Part model, mm, in its own coordinate system. Round coordinates to 2 decimals unless told otherwise and drop trailing zeros. Loops run counter-clockwise (first coordinate to the right, second up) from the corner with the lowest first, then second, coordinate; pieces in that order, holes last.
(1) Cut at A-A on z = 264.5. List the corners of the cut face in (x, y), then the cut area to 3 significant figures.
(2) Probe probe 1 along Y at (x, z) = (-6.9, 186); probe 2 along X at (y, z) = (-2.75, 123); probe 3 along X at (y, z) = (-3, 174.5). List the from-to ranges inside material, lowest first.
(3) Mould opens along X. For faces 1 (the face through (6, 4.95, 148)), 2 (the face through (0, -1.35, 148)), 3 (the face through (9.9, 0, 148)) say: +X half, -X half, draft (parallel to the pull), parting line (faces both ways), or undercut.
(4) Flat gauge pins, fed straight in: pin 1 (4 mm diameter, centred on x = 0, z = 125, fed in from +Y); pin 2 (0.5 mm diameter, centred on y = 5, z = 130, fed in from -X). Where does each tip first touch, or does it go through?
from build123d import *

# Parameters (mm, degrees)
SKETCH_1_R      = 2.1
EXTRUDE_1_DEPTH = 300


with BuildPart() as part:
    # 草图1 → 凸台-拉伸1 (new body)
    with BuildSketch(Plane.XY):
        with BuildLine():
            Line((8.4, -4.95), (-8.4, -4.95))
            ThreePointArc((-8.4, -4.95), (-9.460660172, -4.510660172), (-9.9, -3.45))
            Line((-9.9, -3.45), (-9.9, 3.45))
            ThreePointArc((-9.9, 3.45), (-9.460660172, 4.510660172), (-8.4, 4.95))
            Line((-8.4, 4.95), (-3.5, 4.95))
            Line((-3.5, 4.95), (-3.5, 4.338498403))
            Line((-3.5, 4.338498403), (-3.2, 4.338498403))
            Line((-3.2, 4.338498403), (-3.2, 3.15))
            Line((-3.2, 3.15), (-6.074788311, 3.15))
            Line((-6.074788311, 3.15), (-6.074788311, 0.842971246))
            Line((-6.074788311, 0.842971246), (-2.616641346, -1.35))
            Line((-2.616641346, -1.35), (2.616641346, -1.35))
            Line((2.616641346, -1.35), (6.074788311, 0.842971246))
            Line((6.074788311, 0.842971246), (6.074788311, 3.15))
            Line((6.074788311, 3.15), (3.2, 3.15))
            Line((3.2, 3.15), (3.2, 4.338498403))
            Line((3.2, 4.338498403), (3.5, 4.338498403))
            Line((3.5, 4.338498403), (3.5, 4.95))
            Line((3.5, 4.95), (8.4, 4.95))
            ThreePointArc((8.4, 4.95), (9.460660172, 4.510660172), (9.9, 3.45))
            Line((9.9, 3.45), (9.9, -3.45))
            ThreePointArc((9.9, -3.45), (9.460660172, -4.510660172), (8.4, -4.95))
        make_face()
        with Locations((-6.9, -1.95)):
            Circle(SKETCH_1_R, mode=Mode.SUBTRACT)
        with Locations(Location((6.9, -1.95, 0), (0, 0, 180))):
            Circle(SKETCH_1_R, mode=Mode.SUBTRACT)
    extrude(amount=EXTRUDE_1_DEPTH)


solid = part.part
Final values:
1. outline: (-9.9, -3.45) arc R1.5 ccw to (-8.4, -4.95) - (8.4, -4.95) arc R1.5 ccw to (9.9, -3.45) - (9.9, 3.45) arc R1.5 ccw to (8.4, 4.95) - (3.5, 4.95) - (3.5, 4.34) - (3.2, 4.34) - (3.2, 3.15) - (6.07, 3.15) - (6.07, 0.84) - (2.62, -1.35) - (-2.62, -1.35) - (-6.07, 0.84) - (-6.07, 3.15) - (-3.2, 3.15) - (-3.2, 4.34) - (-3.5, 4.34) - (-3.5, 4.95) - (-8.4, 4.95) arc R1.5 ccw to (-9.9, 3.45) - close; hole circle Ø4.2 at (-6.9, -1.95); hole circle Ø4.2 at (6.9, -1.95)
1. area: 107 mm2
2. probe 1: y = -4.95 to -4.05, 0.15 to 4.95
2. probe 2: x = -9.9 to -8.84, -4.96 to 4.96, 8.84 to 9.9
2. probe 3: x = -9.9 to -8.72, -5.08 to 5.08, 8.72 to 9.9
3. face 1: draft
3. face 2: undercut
3. face 3: +X half
4. pin 1: stops at y = -1.35
4. pin 2: stops at x = -9.15
